```python
from build123d import *

# Parameters (mm, degrees)
BOSS_EXTRUDE1_DEPTH = 80


with BuildPart() as part:
    # Sketch4 → Boss-Extrude1 (new body, symmetric)
    with BuildSketch(Plane.XY):
        with BuildLine():
            Line((4.8, -20), (17.2, -20))
            ThreePointArc((17.2, -20), (19.179898987, -19.179898987), (20, -17.2))
            Line((20, -17.2), (20, -4.8))
            ThreePointArc((20, -4.8), (19.765685425, -4.234314575), (19.2, -4))
            Line((19.2, -4), (16.190663761, -4))
            ThreePointArc((16.190663761, -4), (15.624978336, -4.234314575), (15.390663761, -4.8))
            Line((15.390663761, -4.8), (15.390663761, -10.2))
            ThreePointArc((15.390663761, -10.2), (14.896810507, -10.939103626), (14.024978336, -10.765685425))
            Line((14.024978336, -10.765685425), (9.40588745, -6.146594539))
            ThreePointArc((9.40588745, -6.146594539), (8.365378244, -4.589362465), (8, -2.752481989))
            Line((8, -2.752481989), (8, 0))
            Line((8, 0), (3.5, 0))
            ThreePointArc((3.5, 0), (2.474873734, -2.474873734), (0, -3.5))
            Line((0, -3.5), (0, -8))
            Line((0, -8), (2.752481989, -8))
            ThreePointArc((2.752481989, -8), (4.589362465, -8.365378244), (6.146594539, -9.40588745))
            Line((6.146594539, -9.40588745), (10.765685425, -14.024978336))
            ThreePointArc((10.765685425, -14.024978336), (10.939103626, -14.896810507), (10.2, -15.390663761))
            Line((10.2, -15.390663761), (4.8, -15.390663761))
            ThreePointArc((4.8, -15.390663761), (4.234314575, -15.624978336), (4, -16.190663761))
            Line((4, -16.190663761), (4, -19.2))
            ThreePointArc((4, -19.2), (4.234314575, -19.765685425), (4.8, -20))
        make_face()
    extrude(amount=BOSS_EXTRUDE1_DEPTH, both=True)

    # Mirror1: part across plane


with BuildPart() as part_1:
    add(part.part)
    add(part.part.mirror(Plane(origin=(0, 0, 0), x_dir=(0, 0, 1), z_dir=(1, 0, 0))))

    # Mirror2: part across plane


with BuildPart() as part_2:
    add(part_1.part)
    add(part_1.part.mirror(Plane.ZX))


solid = part_2.part
```
Here's how the part is built. I have some questions about the finished solid (model axes, mm). A direction names the side the tool comes from. Round coordinates to 2 decimals unless told otherwise and drop trailing zeros. Order: outer loops, then holes, each group sorted by start corner. A loop starts at its lowest first (then second) coordinate and runs counter-clockwise, first axis right, second up. Notation, with made-up numbers: M 50,5 L 97,5 A11 cw 97,26 Z; hole C 10.5,-33 d11. An arc over 180 degrees is marked long. Answer in a Markdown table with one row per item.
Item 1: I'm going to push flat-ended pins straight in: pin 1 (1 mm diameter, centred on x = -4, y = 14, fed in from -Z); pin 2 (1.5 mm diameter, centred on y = 18.5, z = -25.5, fed in from +X); pin 3 (1.5 mm diameter, centred on y = -18.5, z = 35, fed in from -X); pin 4 (1 mm diameter, centred on y = 4.5, z = -24, fed in from +X). Where does each tip first touch, or does it pass through?
A:
| item | result |
|---|---|
| pin 1 | passes through |
| pin 2 | stops at x = 19.95 |
| pin 3 | stops at x = -19.95 |
| pin 4 | stops at x = 20 |
Item 2: Thinking about a two-plate mould opening in X: for faces 5 (the face through (-4, 0, -80)), 6 (the face through (-4.565, -8.355, 1.12)), 7 (the face through (-20, 11, 1)), which applies, +X half, -X half, draft (parallel to the pull), parting line (faces both ways), or undercut?
A:
| item | result |
|---|---|
| face 5 | draft |
| face 6 | undercut |
| face 7 | -X half |
Item 3: Imagine slicing it at A-A, the plane x = -12.5. Write out the boundary of the cut face in (y, z), and give its area (3 significant figures).
A:
| item | result |
|---|---|
| outline | M -20,-80 L -9.24,-80 L -9.24,80 L -20,80 Z; M 9.24,-80 L 20,-80 L 20,80 L 9.24,80 Z |
| area | 3,440 mm2 |
Item 4: For faces 1 (the face through (18, 4, 1)), 2 (the face through (-11.75, 8.49, 1.12)), 3 (the face through (-18, -4, 1)), 4 (the face through (4, 18, 1)), which set-ups out of +Z, -Z, +X, -X, +Y, -Y let a thin tool reach every point of the face, with its end or its side?
A:
| item | result |
|---|---|
| face 1 | +Z, -Z, +X |
| face 2 | +Z, -Z |
| face 3 | +Z, -Z, -X |
| face 4 | +Z, -Z, +Y |
Item 5: If I drill on L1, parallel to X at y = -9, z = 48; L2, parallel to Y at x = -17, z = -38; L3, parallel to X at y = 7, z = -57, over which ranges is the centre line in solid material (lowest first)? Write a range as from..to.
A:
| item | result |
|---|---|
| L1 | x = -20..-15.39, -12.26..-5.69, 5.69..12.26, 15.39..20 |
| L2 | y = -20..-4, 4..20 |
| L3 | x = -20..-15.39, -10.26..10.26, 15.39..20 |
